```python
from build123d import *

# Parameters (mm, degrees)
F0_R = 6.35


with BuildPart() as f2:
    # F2: sweep along a path in F1
    with BuildLine(Plane.YZ) as f2_path:
        Line((0, 0), (-6.35, 0))
        ThreePointArc((-6.35, 0), (-10.8401280605, 1.8598719395), (-12.7, 6.35))
        Line((-12.7, 6.35), (-12.7, 120.65))
        ThreePointArc((-12.7, 120.65), (-10.8401280605, 125.1401280605), (-6.35, 127))
        Line((-6.35, 127), (12.7, 127))
        Line((12.7, 127), (30.6605122421, 109.0394877579))
    # F0 (on Front) → F2 (sweep)
    with BuildSketch(Plane.XZ):
        Circle(F0_R)
    sweep(path=f2_path.line, transition=Transition.RIGHT)


solid = f2.part
```
Design review of the part built by this model. Coordinates are the model's own, in mm. A direction names the side the tool comes from. Coordinates: 2 decimals unless noted, no trailing zeros. Write each loop counter-clockwise with the first axis right and the second up, starting at its lowest first coordinate (ties: lowest second). Pieces come first, ordered by that corner, then holes.
1) To check wall thickness, follow L1, parallel to Z at x = -3.75, y = -2; L2, parallel to Y at x = -2.5, z = 13.5; L3, parallel to Y at x = -5, z = 79.5. State the ranges of each line that lie inside material, in increasing order.
2) Add section C-C (z = 96.5). Write out the cut boundary in (x, y), plus the area to 3 significant figures.
3) Mouldability with a two-part tool opening along Y and no side actions: class faces 3 (the cylindrical face through (2.93, 24.873, 122.794)), 4 (the flat face through (0, 0, 0)), 5 (the cylindrical face through (-1.38, -3.22, -6.2)) as +Y half, -Y half, draft (parallel to the pull), parting line (faces both ways), or undercut.
4) Add section B-B (y = 3.5). Write out the cut boundary in (x, z), plus the area to 3 significant figures.
5) Machinability: for faces 1 (the cylindrical face through (-1.38, -18.9, 64.3)), 2 (the flat face through (-0.09, 30.72, 109.1)), which of the approach directions +Z, -Z, +X, -X, +Y, -Y give a long, thin tool a straight path to every point of the face, cutting with its end or side? Answer none if there is none.
6) Add section A-A (x = 3.25). Write out the cut boundary in (y, z).
7) Insertion check: pin 1 (2 mm diameter, centred on y = -9.5, z = 58.5, fed in from +X); pin 2 (6.5 mm diameter, centred on x = -2, z = 0, fed in from +Y); pin 3 (5 mm diameter, centred on x = -1.5, y = 14.5, fed in from -Z). Each pin has a flat end and moves straight along its axis. Give the tip position at first contact, or say it passes through.
8) Add section D-D (x = -4). Write out the cut boundary in (y, z), plus the area to 3 significant figures.
Check result:
1. L1: z = -5.12 to 5.12, 121.88 to 132.12
1. L2: y = -18.54 to -6.86
1. L3: y = -16.61 to -8.79
2. outline: circle Ø12.7 at (0, -12.7)
2. area: 127 mm2
3. face 3: undercut
3. face 4: +Y half
3. face 5: draft
4. outline: circle Ø12.7 at (0, 127)
4. area: 127 mm2
5. face 1: none
5. face 2: -Z, +X, -X, +Y
6. outline: (-18.16, 6.35) arc R11.81 ccw to (-6.35, -5.46) - (0, -5.46) - (0, 5.46) - (-6.35, 5.46) arc R0.89 cw to (-7.24, 6.35) - (-7.24, 120.65) arc R0.89 cw to (-6.35, 121.54) - (10.44, 121.54) - (26.8, 105.18) - (34.52, 112.9) - (14.96, 132.46) - (-6.35, 132.46) arc R11.81 ccw to (-18.16, 120.65) - close
7. pin 1: stops at x = 5.96
7. pin 2: stops at y = 0
7. pin 3: stops at z = 113.88
8. outline: (-17.63, 6.35) arc R11.28 ccw to (-6.35, -4.93) - (0, -4.93) - (0, 4.93) - (-6.35, 4.93) arc R1.42 cw to (-7.77, 6.35) - (-7.77, 120.65) arc R1.42 cw to (-6.35, 122.07) - (10.66, 122.07) - (27.17, 105.55) - (34.15, 112.53) - (14.74, 131.93) - (-6.35, 131.93) arc R11.28 ccw to (-17.63, 120.65) - close
8. area: 1,830 mm2
